```python
from build123d import *

# Parameters (mm, degrees)
ESBO_O1_W                     = 174
ESBO_O1_H                     = 100
ESBO_O1_R                     = 1.25
RESSALTO_EXTRUS_O1_DEPTH      = 3
FILETE1_R                     = 12
ESBO_O2_R                     = 1.35
ESBO_O2_W                     = 29
ESBO_O2_H                     = 59.5
CORTE_EXTRUS_O1_DEPTH         = 10
CONVERTER_S_LIDO1_OUTLINE_R   = 1.25
CONVERTER_S_LIDO1_OUTLINE_R_2 = 1.35
CONVERTER_S_LIDO1_OUTLINE_W   = 29
CONVERTER_S_LIDO1_OUTLINE_H   = 59.5
CONVERTER_S_LIDO1_DEPTH       = 1


# Read off the part's stored shape, not the designer's step: Converter-Sólido1
with BuildPart() as part:
    # Esboço1 → Ressalto-extrusão1 (new body)
    with BuildSketch(Plane.XY):
        Rectangle(ESBO_O1_W, ESBO_O1_H)
        with Locations((-78, -41)):
            Circle(ESBO_O1_R, mode=Mode.SUBTRACT)
        with Locations((-78, 41)):
            Circle(ESBO_O1_R, mode=Mode.SUBTRACT)
        with Locations((78, 41)):
            Circle(ESBO_O1_R, mode=Mode.SUBTRACT)
        with Locations((78, -41)):
            Circle(ESBO_O1_R, mode=Mode.SUBTRACT)
    extrude(amount=RESSALTO_EXTRUS_O1_DEPTH)

    # Filete1
    filete1_edges = [part.edges().sort_by_distance(p)[0] for p in [
        (87, -50, 1.5),
        (-87, -50, 1.5),
        (-87, 50, 1.5),
        (87, 50, 1.5),
    ]]
    fillet(filete1_edges, radius=FILETE1_R)

    # Esboço2 → Corte-extrusão1 (cut)
    with BuildSketch(Plane.XY.offset(3)):
        with Locations((-59.8, 30.5)):
            Circle(ESBO_O2_R)
        with Locations((-59.8, 8.5)):
            Circle(ESBO_O2_R)
        with Locations((-59.8, -13.5)):
            Circle(ESBO_O2_R)
        with Locations((-25.2, -13.5)):
            Circle(ESBO_O2_R)
        with Locations((-25.2, 8.5)):
            Circle(ESBO_O2_R)
        with Locations((-25.2, 30.5)):
            Circle(ESBO_O2_R)
        with Locations((-53.5, 38.3)):
            Circle(ESBO_O2_R)
        with Locations((-31.5, 38.3)):
            Circle(ESBO_O2_R)
        with Locations((31.5, 38.3)):
            Circle(ESBO_O2_R)
        with Locations((53.5, 38.3)):
            Circle(ESBO_O2_R)
        with Locations((25.2, 30.5)):
            Circle(ESBO_O2_R)
        with Locations((25.2, 8.5)):
            Circle(ESBO_O2_R)
        with Locations((25.2, -13.5)):
            Circle(ESBO_O2_R)
        with Locations((59.8, -13.5)):
            Circle(ESBO_O2_R)
        with Locations((59.8, 8.5)):
            Circle(ESBO_O2_R)
        with Locations((59.8, 30.5)):
            Circle(ESBO_O2_R)
        with Locations((-42.5, 5.75)):
            Rectangle(ESBO_O2_W, ESBO_O2_H)
        with Locations((42.5, 5.75)):
            Rectangle(ESBO_O2_W, ESBO_O2_H)
        with BuildLine():
            Line((7.5, 30.5), (7.5, -13.5))
            ThreePointArc((7.5, -13.5), (0, -21), (-7.5, -13.5))
            Line((-7.5, -13.5), (-7.5, 30.5))
            ThreePointArc((-7.5, 30.5), (0, 38), (7.5, 30.5))
        make_face()
    extrude(amount=-CORTE_EXTRUS_O1_DEPTH, mode=Mode.SUBTRACT)

    # Converter-Sólido1 outline → Converter-Sólido1 (cut)
    with BuildSketch(Plane.XY):
        with BuildLine():
            Line((87, -38), (87, 38))
            ThreePointArc((87, 38), (83.485281374, 46.485281374), (75, 50))
            Line((75, 50), (-75, 50))
            ThreePointArc((-75, 50), (-83.485281374, 46.485281374), (-87, 38))
            Line((-87, 38), (-87, -38))
            ThreePointArc((-87, -38), (-83.485281374, -46.485281374), (-75, -50))
            Line((-75, -50), (75, -50))
            ThreePointArc((75, -50), (83.485281374, -46.485281374), (87, -38))
        make_face()
        with Locations((-78, -41)):
            Circle(CONVERTER_S_LIDO1_OUTLINE_R, mode=Mode.SUBTRACT)
        with Locations((-59.8, -13.5)):
            Circle(CONVERTER_S_LIDO1_OUTLINE_R_2, mode=Mode.SUBTRACT)
        with Locations((-25.2, -13.5)):
            Circle(CONVERTER_S_LIDO1_OUTLINE_R_2, mode=Mode.SUBTRACT)
        with Locations((78, -41)):
            Circle(CONVERTER_S_LIDO1_OUTLINE_R, mode=Mode.SUBTRACT)
        with Locations((25.2, -13.5)):
            Circle(CONVERTER_S_LIDO1_OUTLINE_R_2, mode=Mode.SUBTRACT)
        with Locations((59.8, -13.5)):
            Circle(CONVERTER_S_LIDO1_OUTLINE_R_2, mode=Mode.SUBTRACT)
        with Locations((-59.8, 8.5)):
            Circle(CONVERTER_S_LIDO1_OUTLINE_R_2, mode=Mode.SUBTRACT)
        with Locations((-42.5, 5.75)):
            Rectangle(CONVERTER_S_LIDO1_OUTLINE_W, CONVERTER_S_LIDO1_OUTLINE_H, mode=Mode.SUBTRACT)
        with Locations((-25.2, 8.5)):
            Circle(CONVERTER_S_LIDO1_OUTLINE_R_2, mode=Mode.SUBTRACT)
        with Locations((-59.8, 30.5)):
            Circle(CONVERTER_S_LIDO1_OUTLINE_R_2, mode=Mode.SUBTRACT)
        with Locations((-78, 41)):
            Circle(CONVERTER_S_LIDO1_OUTLINE_R, mode=Mode.SUBTRACT)
        with Locations((-53.5, 38.3)):
            Circle(CONVERTER_S_LIDO1_OUTLINE_R_2, mode=Mode.SUBTRACT)
        with Locations((-25.2, 30.5)):
            Circle(CONVERTER_S_LIDO1_OUTLINE_R_2, mode=Mode.SUBTRACT)
        with Locations((-31.5, 38.3)):
            Circle(CONVERTER_S_LIDO1_OUTLINE_R_2, mode=Mode.SUBTRACT)
        with BuildLine():
            ThreePointArc((-7.5, 30.5), (0, 38), (7.5, 30.5))
            Line((7.5, 30.5), (7.5, -13.5))
            ThreePointArc((7.5, -13.5), (0, -21), (-7.5, -13.5))
            Line((-7.5, -13.5), (-7.5, 30.5))
        make_face(mode=Mode.SUBTRACT)
        with Locations((42.5, 5.75)):
            Rectangle(CONVERTER_S_LIDO1_OUTLINE_W, CONVERTER_S_LIDO1_OUTLINE_H, mode=Mode.SUBTRACT)
        with Locations((25.2, 8.5)):
            Circle(CONVERTER_S_LIDO1_OUTLINE_R_2, mode=Mode.SUBTRACT)
        with Locations((59.8, 8.5)):
            Circle(CONVERTER_S_LIDO1_OUTLINE_R_2, mode=Mode.SUBTRACT)
        with Locations((25.2, 30.5)):
            Circle(CONVERTER_S_LIDO1_OUTLINE_R_2, mode=Mode.SUBTRACT)
        with Locations((31.5, 38.3)):
            Circle(CONVERTER_S_LIDO1_OUTLINE_R_2, mode=Mode.SUBTRACT)
        with Locations((59.8, 30.5)):
            Circle(CONVERTER_S_LIDO1_OUTLINE_R_2, mode=Mode.SUBTRACT)
        with Locations((53.5, 38.3)):
            Circle(CONVERTER_S_LIDO1_OUTLINE_R_2, mode=Mode.SUBTRACT)
        with Locations((78, 41)):
            Circle(CONVERTER_S_LIDO1_OUTLINE_R, mode=Mode.SUBTRACT)
    extrude(amount=CONVERTER_S_LIDO1_DEPTH, mode=Mode.SUBTRACT)


solid = part.part
```
Design review of the part built by this model. Coordinates are the model's own, in mm. A direction names the side the tool comes from. Coordinates: 2 decimals unless noted, no trailing zeros. Order: outer loops, then holes, each group sorted by start corner. A loop starts at its lowest first (then second) coordinate and runs counter-clockwise, first axis right, second up.
1) Take a section at C-C, the plane z = 2.2. State how many separate pieces and enclosed holes the cut face has, and give its area (3 significant figures).
2) Take a section at A-A, the plane y = 17. Give the boundary of the cut face in (x, z), and give its area (3 significant figures).
3) For faces 1 (the cylindrical face through (0, -21, 2)), 2 (the flat face through (-21, 1, 1)), list the 3-axis set-ups (+Z, -Z, +X, -X, +Y, -Y) from which the entire face can be reached by the end or side of a thin tool; tool diameter is ignored.
4) Wall thickness on line 1 along X through (y, z) = (2.5, 2.85); line 2 along Y through (x, z) = (-53.5, 2.25); line 3 along Y through (x, z) = (-59.8, 2.2): over which ranges is each line inside the solid? List them lowest first.
5) Take a section at D-D, the plane x = -1.5. Give the boundary of the cut face in (y, z).
6) Clearance check with a flat-ended pin moving along its axis: pin 1 (2.5 mm diameter, centred on x = -25.2, y = 8.5, fed in from +Z). State where the tip first meets the part, or that it passes through.
7) Take a section at B-B, the plane x = -40. Give the boundary of the cut face in (y, z), and give its area (3 significant figures).
8) Mouldability with a two-part tool opening along X and no side actions: class faces 3 (the cylindrical face through (-83.58, 46.39, 2.01)), 4 (the cylindrical face through (83.39, 46.58, 2.01)), 5 (the cylindrical face through (0, 38, 2)) as +X half, -X half, draft (parallel to the pull), parting line (faces both ways), or undercut.
Returned:
1. separate pieces: 1
1. enclosed holes: 23
1. area: 12,900 mm2
2. outline: (-87, 1) - (-57, 1) - (-57, 3) - (-87, 3) - close; (-28, 1) - (-7.5, 1) - (-7.5, 3) - (-28, 3) - close; (7.5, 1) - (28, 1) - (28, 3) - (7.5, 3) - close; (57, 1) - (87, 1) - (87, 3) - (57, 3) - close
2. area: 202 mm2
3. face 1: +Z, -Z
3. face 2: -Z, +X, -X, +Y, -Y
4. line 1: x = -87 to -57, -28 to -7.5, 7.5 to 28, 57 to 87
4. line 2: y = -50 to -24, 35.5 to 36.95, 39.65 to 50
4. line 3: y = -50 to -14.85, -12.15 to 7.15, 9.85 to 29.15, 31.85 to 50
5. outline: (-50, 1) - (-20.85, 1) - (-20.85, 3) - (-50, 3) - close; (37.85, 1) - (50, 1) - (50, 3) - (37.85, 3) - close
6. pin 1: passes through
7. outline: (-50, 1) - (-24, 1) - (-24, 3) - (-50, 3) - close; (35.5, 1) - (50, 1) - (50, 3) - (35.5, 3) - close
7. area: 81.0 mm2
8. face 3: -X half
8. face 4: +X half
8. face 5: undercut
